```python
from build123d import *

# Parameters (mm, degrees)
SKETCH1_W           = 190
SKETCH1_H           = 40
BOSS_EXTRUDE1_DEPTH = 3.175
SKETCH6_R           = 2.5
CUT_EXTRUDE2_DEPTH  = 195.190835584
BOSS_EXTRUDE2_DEPTH = 3.175


with BuildPart() as part:
    # Sketch1 → Boss-Extrude1 (new body)
    with BuildSketch(Plane.XY):
        with Locations((95, 20)):
            Rectangle(SKETCH1_W, SKETCH1_H)
    extrude(amount=BOSS_EXTRUDE1_DEPTH)

    # Sketch6 → Cut-Extrude2 (cut, through all)
    with BuildSketch(Plane.XY.offset(3.175)):
        with Locations((3, 37)):
            Circle(SKETCH6_R)
        with Locations((3, 3)):
            Circle(SKETCH6_R)
        with Locations((187, 37)):
            Circle(SKETCH6_R)
        with Locations((187, 3)):
            Circle(SKETCH6_R)
    extrude(amount=-CUT_EXTRUDE2_DEPTH, mode=Mode.SUBTRACT)

    # Sketch8 → Boss-Extrude2 (add)
    with BuildSketch(Plane.XY.offset(3.175)):
        Polygon((180, -23), (185.764662443, -17.360088892), (190, 0), (180, 0), align=None)
    extrude(amount=-BOSS_EXTRUDE2_DEPTH)


solid = part.part
```
Input: part model. Units: mm. Frame: model coordinates. A direction names the side the tool comes from. Give positions to 0.01 mm unless a question says otherwise; leave off trailing zeros. Order: outer loops, then holes, each group sorted by start corner. A loop starts at its lowest first (then second) coordinate and runs counter-clockwise, first axis right, second up.
1. Cut plane A-A (x = 3). Return loops of the section in (y, z) (3 decimals).
Computed:
outline: (0, 0) - (0.5, 0) - (0.5, 3.175) - (0, 3.175) - close; (5.5, 0) - (34.5, 0) - (34.5, 3.175) - (5.5, 3.175) - close; (39.5, 0) - (40, 0) - (40, 3.175) - (39.5, 3.175) - close
2. Cut plane C-C (y = 37). Return loops of the section in (x, z) (3 decimals).
Computed:
outline: (0, 0) - (0.5, 0) - (0.5, 3.175) - (0, 3.175) - close; (5.5, 0) - (184.5, 0) - (184.5, 3.175) - (5.5, 3.175) - close; (189.5, 0) - (190, 0) - (190, 3.175) - (189.5, 3.175) - close
3. Cut plane D-D (x = 163.5). Return loops of the section in (y, z) (3 decimals), and give its area (3 significant figures).
Computed:
outline: (0, 0) - (40, 0) - (40, 3.175) - (0, 3.175) - close
area: 127 mm2
4. Pin query (flat end, axial travel): pin 1 Ø1.6 at (x, z) = (45, 2) entering from -Y. Return the tip coordinate at first contact, or that it passes through.
Computed:
pin 1: stops at y = 0
5. Set-up query: faces 1 (the face through (89, 0, 2)), 2 (the face through (190, 20, 2)). Return all of +Z, -Z, +X, -X, +Y, -Y with unobstructed straight access to the full face (end or side cutting, diameter ignored); none if empty.
Computed:
face 1: +Z, -Z, -X, -Y
face 2: +Z, -Z, +X, +Y, -Y
6. Line query: probe 1 along Y at (x, z) = (3, 1.4); probe 2 along Y at (x, z) = (37.5, 0.1); probe 3 along X at (y, z) = (-6, 0.95). Output: solid intervals per line, ascending.
Computed:
probe 1: y = 0 to 0.5, 5.5 to 34.5, 39.5 to 40
probe 2: y = 0 to 40
probe 3: x = 180 to 188.54
7. Cut plane B-B (z = 1.75). Return loops of the section in (x, y).
Computed:
outline: (0, 0) - (180, 0) - (180, -23) - (185.76, -17.36) - (190, 0) - (190, 40) - (0, 40) - close; hole circle Ø5 at (3, 3); hole circle Ø5 at (3, 37); hole circle Ø5 at (187, 3); hole circle Ø5 at (187, 37)
